```python
from build123d import *

# Parameters (mm, degrees)
SKETCH1_R               = 12.5
SKETCH1_R_2             = 10.05
BOSS_EXTRUDE1_DEPTH     = 20
SKETCH3_R               = 1.65
CUT_EXTRUDE1_DEPTH      = 4
CIRPATTERN1_COUNT       = 3
SKETCH5_R               = 3
CUT_EXTRUDE3_DEPTH      = 1
CIRPATTERN2_COUNT       = 3
CUT_EXTRUDE5_DEPTH      = 35.369317885
CUT_EXTRUDE5_DEPTH_BACK = 35.369317885
SKETCH7_R               = 1.65
SKETCH8_R               = 3
CUT_EXTRUDE6_DEPTH      = 1
CIRPATTERN6_COUNT       = 2


with BuildPart() as part:
    # Sketch1 → Boss-Extrude1 (new body)
    with BuildSketch(Plane.XY):
        Circle(SKETCH1_R)
        Circle(SKETCH1_R_2, mode=Mode.SUBTRACT)
    extrude(amount=BOSS_EXTRUDE1_DEPTH)

    # Sketch3 → Cut-Extrude1 (cut)
    with BuildSketch(Plane(origin=(-10.825317547, -6.25, 0), x_dir=(0, 0, 1), z_dir=(-0.8660254037844362, -0.5000000000000046, 0))):
        with Locations(Location((4, 0, 0), (0, 0, 270))):
            Circle(SKETCH3_R)
    cut_extrude1 = extrude(amount=-CUT_EXTRUDE1_DEPTH, mode=Mode.SUBTRACT)

    # CirPattern1: Cut-Extrude1 ×3 about axis
    cirpattern1_axis = Axis((0, 0, 0), (0, 0, 1))
    for i in range(1, CIRPATTERN1_COUNT):
        add(cut_extrude1.rotate(cirpattern1_axis, i * 360 / CIRPATTERN1_COUNT), mode=Mode.SUBTRACT)

    # Sketch5 → Cut-Extrude3 (cut)
    with BuildSketch(Plane(origin=(-10.825317547, -6.25, 0), x_dir=(0, 0, 1), z_dir=(-0.8660254037844362, -0.5000000000000046, 0))):
        with Locations(Location((4, 0, 0), (0, 0, 270))):
            Circle(SKETCH5_R)
    cut_extrude3 = extrude(amount=-CUT_EXTRUDE3_DEPTH, mode=Mode.SUBTRACT)

    # CirPattern2: Cut-Extrude3 ×3 about axis
    cirpattern2_axis = Axis((0, 0, 0), (0, 0, 1))
    for i in range(1, CIRPATTERN2_COUNT):
        add(cut_extrude3.rotate(cirpattern2_axis, i * 360 / CIRPATTERN2_COUNT), mode=Mode.SUBTRACT)

    # Sketch7 → Cut-Extrude5 (cut, two sides: drawn at the far end of the back side and taken through both)
    with BuildSketch(Plane.ZY.offset(12.5).offset(-CUT_EXTRUDE5_DEPTH_BACK)):
        with Locations((15, 0)):
            Circle(SKETCH7_R)
    extrude(amount=CUT_EXTRUDE5_DEPTH + CUT_EXTRUDE5_DEPTH_BACK, mode=Mode.SUBTRACT)

    # Sketch8 → Cut-Extrude6 (cut)
    with BuildSketch(Plane.ZY.offset(12.5)):
        with Locations((15, 0)):
            Circle(SKETCH8_R)
    cut_extrude6 = extrude(amount=-CUT_EXTRUDE6_DEPTH, mode=Mode.SUBTRACT)

    # CirPattern6: Cut-Extrude6 ×2 about axis
    cirpattern6_axis = Axis((0, 0, 20), (0, 0, -1))
    for i in range(1, CIRPATTERN6_COUNT):
        add(cut_extrude6.rotate(cirpattern6_axis, i * 360 / CIRPATTERN6_COUNT), mode=Mode.SUBTRACT)


solid = part.part
```
Verification items for the finished model (mm, model axes). A direction names the side the tool comes from. Coordinates: 2 decimals unless noted, no trailing zeros. Loops run counter-clockwise (first coordinate to the right, second up) from the corner with the lowest first, then second, coordinate; pieces in that order, holes last. Notation, with made-up numbers: (81, -1.75) -> (128, -1.75) arc R18 ccw to (128, 14.25) -> close; hole circle Ø8 at (69, 89). An arc over 180 degrees is marked (long way). Answer in a Markdown table with one row per item.
1) Section check D-D (y = 7.75). Record the cut outline in (x, z), and give its area (3 significant figures).
The answers:
| item | result |
|---|---|
| outline | (-9.81, 0) -> (-6.4, 0) -> (-6.4, 20) -> (-9.81, 20) -> close; (6.4, 0) -> (9.81, 0) -> (9.81, 20) -> (6.4, 20) -> close |
| area | 136 mm2 |
2) Section check A-A (y = 0). Record the cut outline in (x, z).
The answers:
| item | result |
|---|---|
| outline | (-12.5, 0) -> (-10.05, 0) -> (-10.05, 13.35) -> (-11.5, 13.35) -> (-11.5, 12) -> (-12.5, 12) -> close; (-12.5, 18) -> (-11.5, 18) -> (-11.5, 16.65) -> (-10.05, 16.65) -> (-10.05, 20) -> (-12.5, 20) -> close; (10.05, 0) -> (12.5, 0) -> (12.5, 12) -> (11.5, 12) -> (11.5, 13.35) -> (10.05, 13.35) -> close; (10.05, 16.65) -> (11.5, 16.65) -> (11.5, 18) -> (12.5, 18) -> (12.5, 20) -> (10.05, 20) -> close |
3) Section check C-C (z = 6). Record the cut outline in (x, y), and give its area (3 significant figures).
The answers:
| item | result |
|---|---|
| outline | (-11.77, -4.21) -> (-11.08, -3.81) -> (-8.84, -7.69) -> (-9.53, -8.09) arc R12.5 ccw to (9.53, -8.09) -> (8.84, -7.69) -> (11.08, -3.81) -> (11.77, -4.21) arc R12.5 ccw to (2.24, 12.3) -> (2.24, 11.5) -> (-2.24, 11.5) -> (-2.24, 12.3) arc R12.5 ccw to start; hole circle Ø20.1 at (0, 0) |
| area | 161 mm2 |
4) Scan lines: line 1 along Z through (x, y) = (0, 11.1); line 2 along Z through (x, y) = (10.45, 0); line 3 along X through (y, z) = (10.75, 2.75). Record each from-to range of solid material in increasing order. Write a range as from..to.
The answers:
| item | result |
|---|---|
| line 1 | z = 0..2.35, 5.65..20 |
| line 2 | z = 0..13.35, 16.65..20 |
| line 3 | x = -6.38..-1.08, 1.08..6.38 |
5) Section check B-B (x = -4.5). Record the cut outline in (y, z), and give its area (3 significant figures).
The answers:
| item | result |
|---|---|
| outline | (-11.66, 0) -> (-8.99, 0) -> (-8.99, 20) -> (-11.66, 20) -> close; (8.99, 0) -> (11.66, 0) -> (11.66, 20) -> (8.99, 20) -> close |
| area | 107 mm2 |
6) Access from +Z, -Z, +X, -X, +Y, -Y to the whole of each face (thin tool, end or side, straight path). Record for faces 1 (the face through (10.605, -4.632, 2.709)), 2 (the face through (11.5, 1.3, 16.3)), 3 (the face through (3, 11.9, 4.1)).
The answers:
| item | result |
|---|---|
| face 1 | none |
| face 2 | +X |
| face 3 | +Y |
7) Depth check by flat-ended pin: P1, Ø4.5, axis at y = 0, z = 15, coming from the +X side; P2, Ø1.8, axis at x = 0, z = 4, coming from the +Y side; P3, Ø3, axis at y = 6, z = 3, coming from the +X side. Enter the tip coordinate at first touch or a pass-through.
The answers:
| item | result |
|---|---|
| P1 | stops at x = 11.5 |
| P2 | stops at y = -10.01 |
| P3 | stops at x = 11.66 |
8) Draft check along Z on faces 4 (the face through (-1.3, 11.5, 2.7)), 5 (the face through (8.46, -6.79, 4.07)), 6 (the face through (0.9, 10.2, 20)), 7 (the face through (0.9, 10.2, 0)). Enter one of: released by +Z, released by -Z, zero draft, split by the parting line, or undercut.
The answers:
| item | result |
|---|---|
| face 4 | undercut |
| face 5 | undercut |
| face 6 | released by +Z |
| face 7 | released by -Z |
